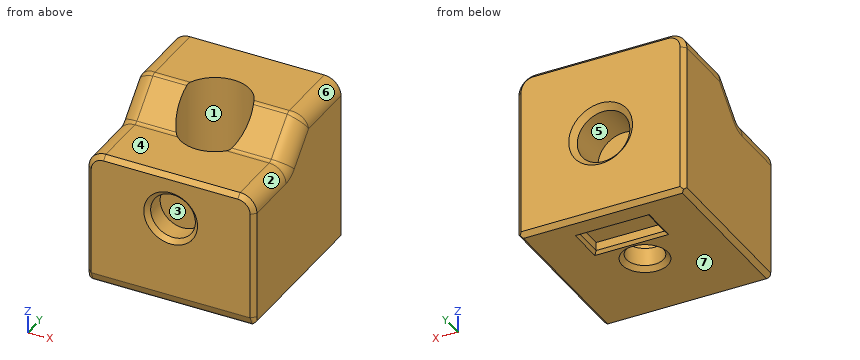
Autodesk Fusion 360 part; units mm, degrees
sketch "Sketch1" plane through (0, 0, 0) normal (0, 0, 1) x (1, 0, 0)
  line L0 (7.5, 7.5) -> (-7.5, 7.5)
  line L1 (-7.5, 7.5) -> (-7.5, -7.5)
  line L2 (-7.5, -7.5) -> (7.5, -7.5)
  line L3 (7.5, -7.5) -> (7.5, 7.5)
  line L4 (7.5, 7.5) -> (-7.5, -7.5) construction
  line L5 (-7.5, 7.5) -> (7.5, -7.5) construction
  circle A0 centre (0, 0) radius 1.65
  circle A1 centre (0, 0) radius 3.1
  dimension "d1" = 15
  dimension "d2" = 15
  dimension "d3" = 3.3
  dimension "d9" = 6.2
extrude "Extrude1" add sketch "Sketch1" along normal blind 15 contours L0 L1 L2 L3 | A1
sketch "Sketch2" plane through (0, 7.5, 0) normal (0, 1, 0) x (-1, 0, 0)
  line L0 (-7.5, 0) -> (7.5, 0)
  line L1 (7.5, 0) -> (7.5, 15)
  line L2 (7.5, 15) -> (-7.5, 15)
  line L3 (-7.5, 15) -> (-7.5, 0)
  circle A0 centre (0, 7.5) radius 2.35
  dimension "d6" = 4.7
extrude "Extrude2" cut sketch "Sketch2" against normal blind 4 contours A0
sketch "Sketch3" plane through (0, 0, 15) normal (0, 0, 1) x (1, 0, 0)
  circle A0 centre (0, 0) radius 1.65
  line L0 (7.5, -7.5) -> (7.5, 7.5)
  line L1 (7.5, 7.5) -> (-7.5, 7.5)
  line L2 (-7.5, 7.5) -> (-7.5, -7.5)
  line L3 (-7.5, -7.5) -> (7.5, -7.5)
  circle A1 centre (0, 0) radius 3.1
extrude "Extrude3" cut sketch "Sketch3" against normal blind 13 contours A1
sketch "Sketch4" plane through (-7.5, 0, 0) normal (-1, 0, 0) x (0, 0, 1)
  line L0 (0, 7.5) -> (0, -7.5)
  line L1 (0, -7.5) -> (15, -7.5)
  line L2 (15, -7.5) -> (15, 7.5)
  line L3 (15, 7.5) -> (0, 7.5)
  line L4 (15, 1) -> (12, -2)
  line L5 (0, -7.5) -> (12, -7.5)
  line L6 (15, 1) -> (15, 7.5)
  line L7 (5.15, 3.5) -> (9.85, 3.5)
  line L8 (5.15, 7.5) -> (9.85, 7.5)
  line L9 (12, -4) -> (0, -4)
  line L10 (12, -2) -> (12, -4)
  line L11 (12, -4) -> (12, -7.5)
  dimension "d12" = 12
  dimension "d20" = 3
  dimension "d21" = 3.5
  dimension "d22" = 135
  dimension "d23" = 5.5
extrude "Extrude4" cut sketch "Sketch4" against normal blind 186 contours L1 L2 L4 L10 L11
fillet "Fillet1" radius 0.5 4 edges at (-5.2171, 1, 15) (5.2171, 1, 15) (4.9343, -2, 12) (-4.9343, -2, 12)
fillet "Fillet2" radius 1.5 10 edges at (7.5, 4.3536, 15) (7.5, 1.0158, 14.9619) (7.5, -0.5, 13.5) (7.5, -2.0158, 12.0381) (7.5, -4.8536, 12) (-7.5, 4.3536, 15) (-7.5, 1.0158, 14.9619) (-7.5, -0.5, 13.5) (-7.5, -2.0158, 12.0381) (-7.5, -4.8536, 12)
chamfer "Chamfer2" distance 0.5 angle 45 1 edges at (2.191, 7.5, 8.3498)
chamfer "Chamfer1" distance 0.4 angle 45 1 faces at (0.0411, -5.5485, 0)
chamfer "Chamfer3" distance 0.4 angle 45 1 faces at (2, -7.5, 4.2667)
sketch "Sketch5" plane through (0, -7.5, 0) normal (0, -1, 0) x (1, 0, 0)
  line L0 (7.1, 0.8) -> (7.1, 10.5)
  line L1 (-7.1, 10.5) -> (-7.1, 0.8)
  line L2 (-7.1, 0.8) -> (7.1, 0.8)
  circle A0 centre (0, 8) radius 2
  line L3 (-7.1, 0) -> (7.1, 0)
  arc A1 (7.1, 10.5) -> (6, 11.6) centre (6, 10.5) ccw
  line L4 (6, 11.6) -> (-6, 11.6)
  arc A2 (-6, 11.6) -> (-7.1, 10.5) centre (-6, 10.5) ccw
  line L5 (6, 12) -> (-6, 12)
  dimension "d28" = 8
  dimension "d29" = 4
  dimension "d34" = 4
extrude "Extrude5" cut sketch "Sketch5" against normal blind 2 contours A0
chamfer "Chamfer4" distance 0.4 angle 45 6 edges at (-1.8647, -7.5, 8.7232) (7.5, 7.5, 6.95) (7.0607, 7.5, 14.5607) (0, 7.5, 15) (-7.0607, 7.5, 14.5607) (-7.5, 7.5, 6.95)
sketch "Sketch6" plane through (0, 0, 0) normal (0, 0, -1) x (-1, 0, 0)
  circle A0 centre (0, 0) radius 2.05
  line L0 (-7.1, 7.1) -> (-7.1, -7.1)
  line L1 (-7.1, -7.1) -> (7.1, -7.1)
  line L2 (7.1, -7.1) -> (7.1, 7.1)
  line L3 (7.1, 7.1) -> (-7.1, 7.1)
  line L4 (-3.041, 5.3) -> (3.059, 5.3)
  line L5 (3.059, 5.3) -> (3.059, 2.5)
  line L6 (3.059, 2.5) -> (-3.041, 2.5)
  line L7 (-3.041, 2.5) -> (-3.041, 5.3)
  line L8 (-7.5, 7.1) -> (-7.5, -7.1)
  line L9 (7.1, 7.5) -> (-7.1, 7.5)
  dimension "d35" = 6.1
  dimension "d36" = 2.8
  dimension "d37" = 4.459
  dimension "d38" = 2.2
extrude "Extrude6" cut sketch "Sketch6" against normal blind 1 contours L4 L5 L6 L7
chamfer "Chamfer5" distance 0.25 angle 45 4 edges at (-3.059, 3.9, 0) (-0.009, 5.3, 0) (-0.009, 2.5, 0) (3.041, 3.9, 0)
equation "d10 = -15 mm + 2 mm"
Verification items for the finished model (mm, model axes). Face numbers are marked on the shaded views. A direction names the side the tool comes from. Give positions to 0.01 mm unless a question says otherwise; leave off trailing zeros. Write each loop counter-clockwise with the first axis right and the second up, starting at its lowest first coordinate (ties: lowest second). Pieces come first, ordered by that corner, then holes. Notation, with made-up numbers: M 20.25,-38 L 30.25,-38 A26 ccw 30.25,-20 Z; hole C -28.75,-30.75 d7. An arc over 180 degrees is marked long. Put each result on its own line as item: value. Start each with the question number.
1. Section check A-A (z = 1.5). Record the cut outline in (x, y), and give its area (3 significant figures).
2. Section check B-B (x = 3.75). Record the cut outline in (y, z).
3. Scan lines: line 1 along Z through (x, y) = (0, 5.9); line 2 along Z through (x, y) = (0, 5.1); line 3 along Z through (x, y) = (5, -4.5). Record each from-to range of solid material in increasing order. Write a range as [from, to].
4. Draft check along Z on the marked faces 5, 6 and 7. Enter one of: +Z half, -Z half, draft (parallel to the pull), parting line (faces both ways), or undercut.
5. Section check C-C (z = 4.25). Record the cut outline in (x, y), and give its area (3 significant figures).
6. Set-up check for the marked faces 1, 2, 3 and 4: record each of +Z, -Z, +X, -X, +Y, -Y from which the full face is reachable in a straight line by a thin tool's end or side.
7. Go/stop test with flat-tipped pins: pin 1 Ø3 at (x, z) = (0, 7.5) entering from +Y; pin 2 Ø5.5 at (x, y) = (-0.5, -4) entering from +Z; pin 3 Ø3 at (x, y) = (0, 4) entering from -Z. Record where each tip stops, or that it passes through.
Answer list:
1. outline: M -7.5,-7.1 L -7.1,-7.5 L 7.1,-7.5 L 7.5,-7.1 L 7.5,7.1 L 7.1,7.5 L -7.1,7.5 L -7.5,7.1 Z; hole C 0,0 d3.3
1. area: 216 mm2
2. outline: M -7.5,0.8 L -7.22,0.12 L -7.1,0 L 7.1,0 L 7.5,0.4 L 7.5,14.6 L 7.1,15 L 1.21,15 A0.5 ccw 0.85,14.85 L -1.85,12.15 A0.5 cw -2.21,12 L -7.1,12 L -7.5,11.6 Z
3. line 1: [0, 5.15], [9.85, 15]
3. line 2: [1, 5.15], [9.85, 15]
3. line 3: [0, 12]
4. face 5: undercut
4. face 6: +Z half
4. face 7: -Z half
5. outline: M -7.5,-7.1 L -7.1,-7.5 L 7.1,-7.5 L 7.5,-7.1 L 7.5,7.1 L 7.1,7.5 L -7.1,7.5 L -7.5,7.1 Z; hole C 0,0 d6.2
5. area: 194 mm2
6. face 1: +Z
6. face 2: +Z, +X, -Y
6. face 3: -Y
6. face 4: +Z, +X, -X, -Y
7. pin 1: y = 3.5
7. pin 2: z = 12.05
7. pin 3: z = 0.05
